```python
from build123d import *

# Parameters (mm, degrees)
SKETCH_1_R       = 2.7
SKETCH_1_R_2     = 2.2
EXTRUDE_1_DEPTH  = 5
SKETCH_1_4_W     = 29.617054823
SKETCH_1_4_H     = 2
EXTRUDE_2_DEPTH  = 6.8
CHAMFER_1_SIZE   = 3
CHAMFER_1_SIZE_2 = 6.8
CHAMFER_2_SIZE   = 3
CHAMFER_2_SIZE_2 = 6.8


with BuildPart() as part:
    # 草图1 → 凸台-拉伸1 (new body)
    with BuildSketch(Plane.XY):
        with BuildLine():
            Line((-22.196745644, 31.383682827), (-46.231163763, 8.922455218))
            ThreePointArc((-46.231163763, 8.922455218), (-47.169104458, 7.593007368), (-47.5, 6))
            Line((-47.5, 6), (-47.5, -6))
            ThreePointArc((-47.5, -6), (-47.169104458, -7.593007368), (-46.231163763, -8.922455218))
            Line((-46.231163763, -8.922455218), (-22.196745644, -31.383682827))
            ThreePointArc((-22.196745644, -31.383682827), (-19.384432728, -32.860907145), (-16.212075635, -32.695238502))
            Line((-16.212075635, -32.695238502), (19.987924365, -20.695238502))
            ThreePointArc((19.987924365, -20.695238502), (22.964542434, -18.512296529), (24.1, -15))
            Line((24.1, -15), (24.1, 15))
            ThreePointArc((24.1, 15), (22.964542434, 18.512296529), (19.987924365, 20.695238502))
            Line((19.987924365, 20.695238502), (-16.212075635, 32.695238502))
            ThreePointArc((-16.212075635, 32.695238502), (-19.384432728, 32.860907145), (-22.196745644, 31.383682827))
        make_face()
        with Locations((18.1, -15)):
            Circle(SKETCH_1_R, mode=Mode.SUBTRACT)
        with Locations((-38, 0)):
            Circle(SKETCH_1_R_2, mode=Mode.SUBTRACT)
        with Locations((-18, 0)):
            Circle(SKETCH_1_R_2, mode=Mode.SUBTRACT)
        with Locations((-18.1, 27)):
            Circle(SKETCH_1_R, mode=Mode.SUBTRACT)
        with Locations((18.1, 15)):
            Circle(SKETCH_1_R, mode=Mode.SUBTRACT)
        with Locations((-18.1, -27)):
            Circle(SKETCH_1_R, mode=Mode.SUBTRACT)
    extrude(amount=EXTRUDE_1_DEPTH)

    # 草图4 → 旋转1 (revolve)
    with BuildSketch(Plane(origin=(6.272104728, 18.920849262, 0), x_dir=(-0.9492064169502825, 0.3146540608674969, 0), z_dir=(-0.3146540608674969, -0.9492064169502825, 0)), mode=Mode.PRIVATE) as revolve_1_sk:
        Polygon((-6.460825234, 0), (-7.460825234, 8.7), (-9.760825234, 8.7), (-9.760825234, 0), align=None)
    revolve_1 = revolve(revolve_1_sk.sketch.rotate(Axis((18.1, 15, 4.45283877), (0, 0, -1)), 161.660068966), axis=Axis((18.1, 15, 4.45283877), (0, 0, -1)))

    # 草图4<3> → 旋转2 (revolve)
    with BuildSketch(Plane(origin=(6.272104728, 18.920849262, 0), x_dir=(-0.9492064169502825, 0.3146540608674969, 0), z_dir=(-0.3146540608674969, -0.9492064169502825, 0)), mode=Mode.PRIVATE) as revolve_2_sk:
        Polygon((30.67629579, 8.7), (28.37629579, 8.7), (28.37629579, 0), (31.67629579, 0), align=None)
    revolve_2 = revolve(revolve_2_sk.sketch.rotate(Axis((-18.1, 27, 0), (0, 0, -1)), 161.660068966), axis=Axis((-18.1, 27, 0), (0, 0, -1)))

    # 镜向1: 旋转1, 旋转2 across plane
    add(revolve_1.mirror(Plane.ZX))
    add(revolve_2.mirror(Plane.ZX))

    # 草图1<4> → 凸台-拉伸2 (add)
    with BuildSketch(Plane.XY):
        with Locations((-27.808527412, 11.3)):
            Rectangle(SKETCH_1_4_W, SKETCH_1_4_H)
        with Locations((-27.808527412, -11.3)):
            Rectangle(SKETCH_1_4_W, SKETCH_1_4_H)
    extrude(amount=-EXTRUDE_2_DEPTH)

    # 倒角1
    # the kernel refuses this chamfer: 6.8, 3 mm, written as the material it adds along each edge
    with BuildSketch(Plane(origin=(-13, 12.3, 0), x_dir=(0, 0.9968133817371192, 0.07976892872421078), z_dir=(-1, 0, 0))) as chamfer_1_piece_1_section:
        Polygon((CHAMFER_1_SIZE * 0.996813381737, CHAMFER_1_SIZE * 0.0797689287242), (-CHAMFER_1_SIZE_2 * 0.0797689287242, CHAMFER_1_SIZE_2 * 0.996813381737), (0, 0), align=None)
    chamfer_1_piece_1 = extrude(amount=29.617054823, mode=Mode.PRIVATE)
    chamfer_1_piece_1 = split(chamfer_1_piece_1, bisect_by=Plane(origin=(-33.986119971, 20.365990665, -2.314362064), z_dir=(0.6827909407070696, -0.730613804474262, 0)), keep=Keep.TOP, mode=Mode.PRIVATE)
    chamfer_1_piece_1 = split(chamfer_1_piece_1, bisect_by=Plane(origin=(-27.310795563, 13.223124714, -6.8), z_dir=(0, 0, 1)), keep=Keep.TOP, mode=Mode.PRIVATE)
    add(chamfer_1_piece_1)

    # 倒角2
    # the kernel refuses this chamfer: 6.8, 3 mm, written as the material it adds along each edge
    with BuildSketch(Plane(origin=(-42.617054823, -12.3, 0), x_dir=(0, -0.9968133817371192, 0.07976892872421078), z_dir=(1, 0, 0))) as chamfer_2_piece_1_section:
        Polygon((CHAMFER_2_SIZE * 0.996813381737, CHAMFER_2_SIZE * 0.0797689287242), (-CHAMFER_2_SIZE_2 * 0.0797689287242, CHAMFER_2_SIZE_2 * 0.996813381737), (0, 0), align=None)
    chamfer_2_piece_1 = extrude(amount=29.617054823, mode=Mode.PRIVATE)
    chamfer_2_piece_1 = split(chamfer_2_piece_1, bisect_by=Plane(origin=(-33.986119971, -20.365990665, -2.314362064), z_dir=(0.6827909407070697, 0.7306138044742619, 0)), keep=Keep.TOP, mode=Mode.PRIVATE)
    chamfer_2_piece_1 = split(chamfer_2_piece_1, bisect_by=Plane(origin=(-27.310795563, -13.223124714, -6.8), z_dir=(0, 0, 1)), keep=Keep.TOP, mode=Mode.PRIVATE)
    add(chamfer_2_piece_1)


solid = part.part
```
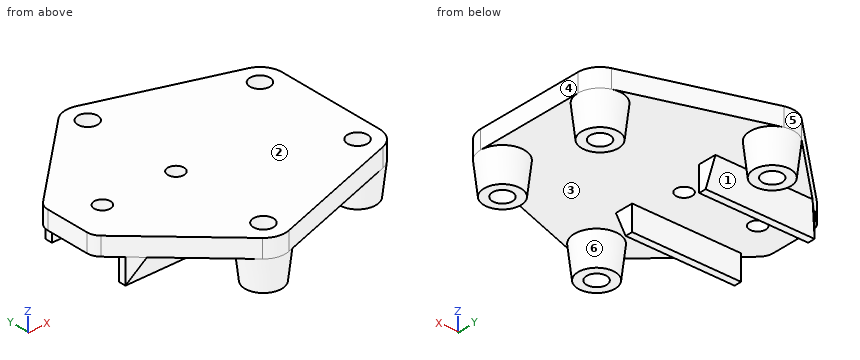
Design review of the part built by this model. Coordinates are the model's own, in mm. Face numbers are marked on the shaded views. A direction names the side the tool comes from. Coordinates: 2 decimals unless noted, no trailing zeros. Loops run counter-clockwise (first coordinate to the right, second up) from the corner with the lowest first, then second, coordinate; pieces in that order, holes last. Notation, with made-up numbers: (10.5, -22) - (44.5, -22) arc R22 ccw to (44.5, -8) - close; hole circle Ø7 at (74, 20.5). An arc over 180 degrees is marked (long way). Use CSV: the item, a comma, the result in double quotes. Start each with the question number.
1) Tool access review of the marked faces 1, 2 and 3: name each direction out of +Z, -Z, +X, -X, +Y, -Y from which nothing blocks a thin tool from reaching the whole face with its end or side.
2) For pin 1 Ø3 at (x, z) = (-15, 1.5) entering from +Y; pin 2 Ø1 at (x, z) = (-12.5, 0.5) entering from +Y; pin 3 Ø5.5 at (x, y) = (-38, 0) entering from +Z; pin 4 Ø1.5 at (x, y) = (12, -22) entering from -Z, all flat-tipped, find the tip position at first contact; note any pin that passes through.
3) The part is to be moulded in two halves that separate along Y. For the marked faces 4, 5 and 6, say which applies: +Y half, -Y half, draft (parallel to the pull), parting line (faces both ways), or undercut.
4) Wall thickness on L1, parallel to Y at x = -18, z = 1.45; L2, parallel to Y at x = 19, z = 3.75; L3, parallel to Y at x = -18.1, z = -5.5: over which ranges is each line inside the solid? List them lowest first. Write a range as from..to.
5) Consider section C-C on y = 27. Write out the cut boundary in (x, z).
6) Consider section A-A on z = -4.75. Give the number of separate pieces and of enclosed holes in the cut face, then the cut area to 3 significant figures.
7) Consider section B-B on z = 2.5. Write out the cut boundary in (x, y), then the cut area to 3 significant figures.
Geometry says:
1,face 1,"-Z, -X"
1,face 2,"+Z, +X, -X, +Y, -Y"
1,face 3,"-Z"
2,pin 1,"y = 32.78"
2,pin 2,"y = 31.63"
2,pin 3,"z = 5"
2,pin 4,"z = 0"
3,face 4,"draft"
3,face 5,"+Y half"
3,face 6,"undercut"
4,L1,"-33..-29.7, -24.3..-2.2, 2.2..24.3, 29.7..33"
4,L2,"-21.02..-17.55, -12.45..12.45, 17.55..21.02"
4,L3,"-32.37..-29.7, -24.3..-21.63, -12.87..-10.3, 10.3..12.87, 21.63..24.3, 29.7..32.37"
5,outline,"(-26.89, 0) - (-24.1, 0) - (-23.1, -8.7) - (-20.8, -8.7) - (-20.8, 5) - (-26.89, 5) - close; (-15.4, -8.7) - (-13.1, -8.7) - (-12.1, 0) - (0.97, 0) - (0.97, 5) - (-15.4, 5) - close"
6,separate pieces,"6"
6,enclosed holes,"4"
6,area,"453 mm^2"
7,outline,"(-47.5, -6) arc R4 ccw to (-46.23, -8.92) - (-22.2, -31.38) arc R6 ccw to (-16.21, -32.7) - (19.99, -20.7) arc R6 ccw to (24.1, -15) - (24.1, 15) arc R6 ccw to (19.99, 20.7) - (-16.21, 32.7) arc R6 ccw to (-22.2, 31.38) - (-46.23, 8.92) arc R4 ccw to (-47.5, 6) - close; hole circle Ø4.4 at (-38, 0); hole circle Ø5.4 at (-18.1, -27); hole circle Ø5.4 at (-18.1, 27); hole circle Ø4.4 at (-18, 0); hole circle Ø5.4 at (18.1, -15); hole circle Ø5.4 at (18.1, 15)"
7,area,"3,350 mm^2"
